Read the model definition and answer for the solid it produces. Units are mm, in the model's axes. A direction names the side the tool comes from. Give positions to 0.01 mm unless a question says otherwise; leave off trailing zeros. Write each loop counter-clockwise with the first axis right and the second up, starting at its lowest first coordinate (ties: lowest second). Pieces come first, ordered by that corner, then holes. Notation, with made-up numbers: (8.5, -9.75) -> (49.5, -9.75) arc R28 ccw to (49.5, 24.25) -> close; hole circle Ø8 at (61.25, 86.25). An arc over 180 degrees is marked (long way). Use a Markdown table: item, result.
from build123d import *

# Parameters (mm, degrees)
SKETCH1_W           = 33
SKETCH1_H           = 13
BOSS_EXTRUDE1_DEPTH = 2
BOSS_EXTRUDE2_DEPTH = 1
FILLET1_R           = 0.5
SKETCH3_R           = 0.631168426
CUT_EXTRUDE1_DEPTH  = 0.1
FILLET2_R           = 0.04
SKETCH4_R           = 0.625
BOSS_EXTRUDE3_DEPTH = 0.6
BOSS_EXTRUDE3_TAPER = 27
SKETCH7_R           = 1
CUT_EXTRUDE2_DEPTH  = 3


with BuildPart() as part:
    # Sketch1 → Boss-Extrude1 (new body)
    with BuildSketch(Plane(origin=(0, 0, 0), x_dir=(1, 0, 0), z_dir=(0, 1, 0))):
        Rectangle(SKETCH1_W, SKETCH1_H)
    extrude(amount=BOSS_EXTRUDE1_DEPTH)

    # Sketch2 → Boss-Extrude2 (add)
    with BuildSketch(Plane(origin=(0, 2, 0), x_dir=(1, 0, 0), z_dir=(0, 1, 0))):
        Polygon((-11.063698409, -0.221797323), (-5.897125464, -4.944775622), (-1.174147166, 0.221797323), (-6.340720111, 4.944775622), align=None)
    extrude(amount=BOSS_EXTRUDE2_DEPTH)

    # Fillet1
    fillet1_edges = [part.edges().sort_by_distance(p)[0] for p in [
        (-8.70220926, 3, -2.361489149),
        (-8.480411937, 3, 2.583286472),
        (-3.535636315, 3, 2.361489149),
        (-3.757433638, 3, -2.583286472),
    ]]
    fillet(fillet1_edges, radius=FILLET1_R)

    # Sketch3 → Cut-Extrude1 (cut)
    with BuildSketch(Plane(origin=(0, 3, 0), x_dir=(1, 0, 0), z_dir=(0, 1, 0))):
        with Locations(Location((-2.868853152, 0.151489879, 0), (0, 0, 270))):
            Circle(SKETCH3_R)
    extrude(amount=-CUT_EXTRUDE1_DEPTH, mode=Mode.SUBTRACT)

    # Fillet2
    fillet2_edges = [part.edges().sort_by_distance(p)[0] for p in [
        (-2.868853152, 3, -0.782658305),
    ]]
    fillet(fillet2_edges, radius=FILLET2_R)

    # Sketch4 → Boss-Extrude3 (add)
    with BuildSketch(Plane(origin=(0, 2, 0), x_dir=(1, 0, 0), z_dir=(0, 1, 0))):
        with Locations((-13.5, 5.5)):
            Circle(SKETCH4_R)
        with Locations((-11.25, 5.5)):
            Circle(SKETCH4_R)
        with Locations((-9, 5.5)):
            Circle(SKETCH4_R)
        with Locations((-6.75, 5.5)):
            Circle(SKETCH4_R)
        with Locations((-4.5, 5.5)):
            Circle(SKETCH4_R)
        with Locations((-2.25, 5.5)):
            Circle(SKETCH4_R)
        with Locations((0, 5.5)):
            Circle(SKETCH4_R)
        with Locations((2.25, 5.5)):
            Circle(SKETCH4_R)
        with Locations((4.5, 5.5)):
            Circle(SKETCH4_R)
        with Locations((6.75, 5.5)):
            Circle(SKETCH4_R)
        with Locations((9, 5.5)):
            Circle(SKETCH4_R)
        with Locations((11.25, 5.5)):
            Circle(SKETCH4_R)
        with Locations((13.5, 5.5)):
            Circle(SKETCH4_R)
        with Locations((-13.5, -5.5)):
            Circle(SKETCH4_R)
        with Locations((-11.25, -5.5)):
            Circle(SKETCH4_R)
        with Locations((-9, -5.5)):
            Circle(SKETCH4_R)
        with Locations((-6.75, -5.5)):
            Circle(SKETCH4_R)
        with Locations((-4.5, -5.5)):
            Circle(SKETCH4_R)
        with Locations((-2.25, -5.5)):
            Circle(SKETCH4_R)
        with Locations((0, -5.5)):
            Circle(SKETCH4_R)
        with Locations((2.25, -5.5)):
            Circle(SKETCH4_R)
        with Locations((4.5, -5.5)):
            Circle(SKETCH4_R)
        with Locations((6.75, -5.5)):
            Circle(SKETCH4_R)
        with Locations((9, -5.5)):
            Circle(SKETCH4_R)
        with Locations((11.25, -5.5)):
            Circle(SKETCH4_R)
        with Locations((13.5, -5.5)):
            Circle(SKETCH4_R)
    extrude(amount=BOSS_EXTRUDE3_DEPTH, taper=BOSS_EXTRUDE3_TAPER)

    # Sketch7 → Cut-Extrude2 (cut)
    with BuildSketch(Plane(origin=(0, 2, 0), x_dir=(1, 0, 0), z_dir=(0, 1, 0))):
        with Locations(Location((15, 2.5, 0), (0, 0, 270))):
            Circle(SKETCH7_R)
    extrude(amount=-CUT_EXTRUDE2_DEPTH, mode=Mode.SUBTRACT)


solid = part.part
Item 1: A cutting plane is placed at A-A (x = 15). Give the vertices of the cut face in (y, z), then the cut area to 3 significant figures.
Return value:
| item | result |
|---|---|
| outline | (0, -6.5) -> (2, -6.5) -> (2, -3.5) -> (0, -3.5) -> close; (0, -1.5) -> (2, -1.5) -> (2, 6.5) -> (0, 6.5) -> close |
| area | 22.0 mm^2 |
Item 2: A cutting plane is placed at B-B (x = 8). Give the vertices of the cut face in (y, z), then the cut area to 3 significant figures.
Return value:
| item | result |
|---|---|
| outline | (0, -6.5) -> (2, -6.5) -> (2, 6.5) -> (0, 6.5) -> close |
| area | 26.0 mm^2 |
Item 3: Each of these flat-tipped pins is pushed along its axis until it touches: P1, Ø0.7, axis at x = 4.5, z = 5.5, coming from the +Y side; P2, Ø2, axis at x = 12, z = -0.5, coming from the +Y side; P3, Ø0.6, axis at x = -3, z = 0, coming from the +Y side. Where does it stop, or does it pass through?
Return value:
| item | result |
|---|---|
| P1 | y = 2.6 |
| P2 | y = 2 |
| P3 | y = 2.9 |
Item 4: Straight lines are drawn through the part: line 1 along X through (y, z) = (0.4, -2.5); line 2 along Y through (x, z) = (3, 2.75); line 3 along X through (y, z) = (0.85, -3.25). For each, find the intervals that lie inside material, in ascending order. Write a range as [from, to].
Return value:
| item | result |
|---|---|
| line 1 | [-16.5, 14], [16, 16.5] |
| line 2 | [0, 2] |
| line 3 | [-16.5, 14.34], [15.66, 16.5] |
Item 5: A tool of negligible diameter and unlimited length cuts with its end or side. For faces 3 (the face through (0, 2, 0)), 4 (the face through (-16.5, 1, 0)), from which of +Z, -Z, +X, -X, +Y, -Y can it reach the whole face along a straight path? Write none if from no direction.
Return value:
| item | result |
|---|---|
| face 3 | +Y |
| face 4 | +Z, -Z, -X, +Y, -Y |
Item 6: For a pull along Z with two mould halves and no side action, classify faces 1 (the face through (0, 0, 0)), 2 (the face through (-3.57, 2.25, 2.4)) as +Z half, -Z half, draft (parallel to the pull), parting line (faces both ways), or undercut.
Return value:
| item | result |
|---|---|
| face 1 | draft |
| face 2 | undercut |
